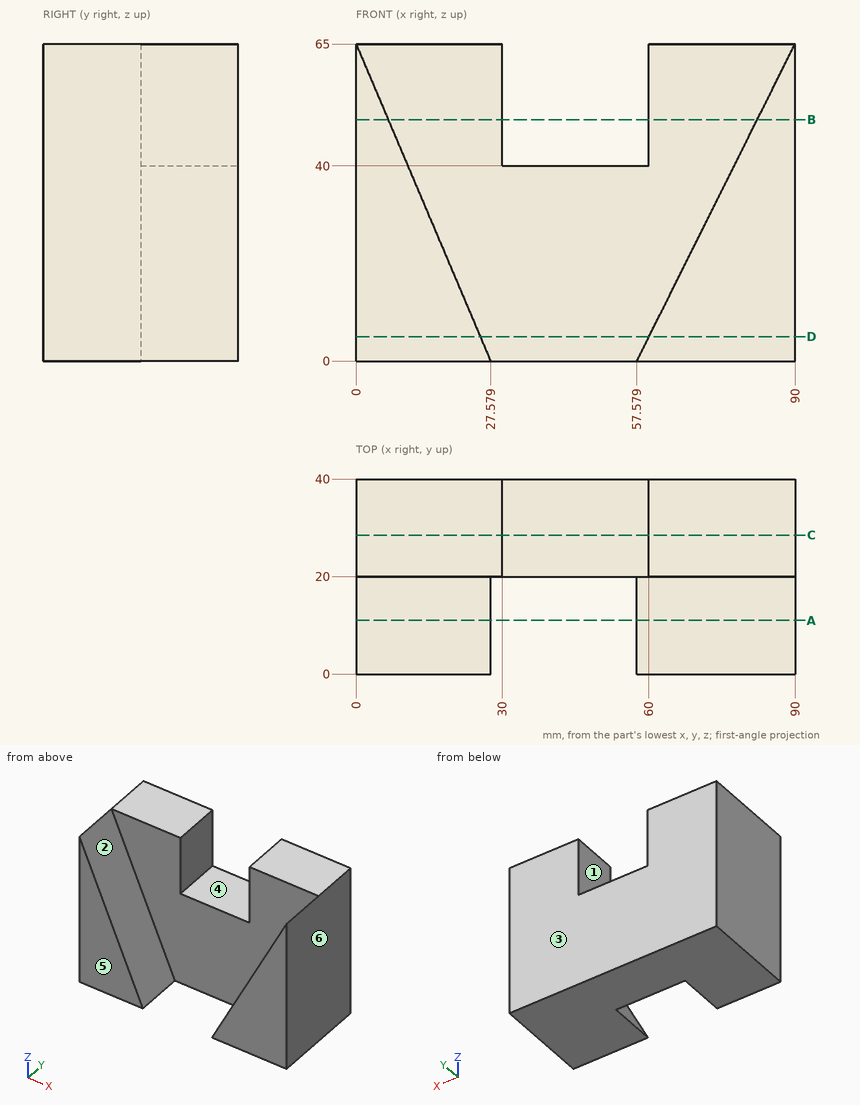
The drawing under review shows one solid part. Ordinate dimensions are in mm from its lowest x, y, z. A direction names the side the tool comes from. Give positions to 0.01 mm unless a question says otherwise; leave off trailing zeros. Order: outer loops, then holes, each group sorted by start corner. A loop starts at its lowest first (then second) coordinate and runs counter-clockwise, first axis right, second up. Notation, with made-up numbers: (8.5, 65.5) - (53.5, 65.5) arc R37 cw to (53.5, 103.5) - close; hole circle Ø8 at (-28, -21.75). An arc over 180 degrees is marked (long way). Answer as a JSON object with one key per item and string values. Group by question number.
Item 1: Draft analysis for pull direction X (two halves, no side actions). For the marked faces 4, 5 and 6, state which applies: pulls with the +X half, pulls with the -X half, needs draft (parallel to the pull), parting line crosses it, or undercut.
Item 2: Take a section at B-B on z = 49.5. Give the boundary of the cut face in (x, y).
Item 3: Wall thickness on line 1 along Z through (x, y) = (50.5, 27.5); line 2 along Y through (x, z) = (61, 57); line 3 along X through (y, z) = (13, 17.5): over which ranges is each line inside the solid? List them lowest first.
Item 4: Take a section at D-D on z = 5. Give the boundary of the cut face in (x, y), and give its area (3 significant figures).
Item 5: Take a section at C-C on y = 28.5. Give the boundary of the cut face in (x, z), and give its area (3 significant figures).
Item 6: Machinability: for the marked faces 1, 2 and 3, which of the approach directions +Z, -Z, +X, -X, +Y, -Y give a long, thin tool a straight path to every point of the face, cutting with its end or side? Answer none if there is none.
Item 7: Take a section at A-A on y = 11. Give the boundary of the cut face in (x, z), and give its area (3 significant figures).
Item 8: Clearance check with flat-ended pins moving along their axes: pin 1 Ø19.5 at (x, z) = (46, 33.5) entering from -Y; pin 2 Ø10 at (x, y) = (21.5, 6.5) entering from +Z; pin 3 Ø10 at (x, y) = (51.5, 35) entering from +Z; pin 4 Ø3 at (x, z) = (57, 45) entering from +Y. State where each tip first meets the part, or that it passes through.
Reported:
{
 "1": {"face 4": "undercut", "face 5": "needs draft", "face 6": "pulls with the +X half"},
 "2": {"outline": "(0, 0) - (6.58, 0) - (6.58, 20) - (30, 20) - (30, 40) - (0, 40) - close; (60, 20) - (82.27, 20) - (82.27, 0) - (90, 0) - (90, 40) - (60, 40) - close"},
 "3": {"line 1": "0 to 40", "line 2": "20 to 40", "line 3": "0 to 20.15, 66.31 to 90"},
 "4": {"outline": "(0, 0) - (25.46, 0) - (25.46, 20) - (60.07, 20) - (60.07, 0) - (90, 0) - (90, 40) - (0, 40) - close", "area": "2,910 mm^2"},
 "5": {"outline": "(0, 0) - (90, 0) - (90, 65) - (60, 65) - (60, 40) - (30, 40) - (30, 65) - (0, 65) - close", "area": "5,100 mm^2"},
 "6": {"face 1": "+Z, +Y, -Y", "face 2": "+Z, -Y", "face 3": "+Z, -Z, +X, -X, +Y"},
 "7": {"outline": "(0, 0) - (27.58, 0) - (0, 65) - close; (57.58, 0) - (90, 0) - (90, 65) - close", "area": "1,950 mm^2"},
 "8": {"pin 1": "y = 20", "pin 2": "z = 26.11", "pin 3": "z = 40", "pin 4": "through"}
}
